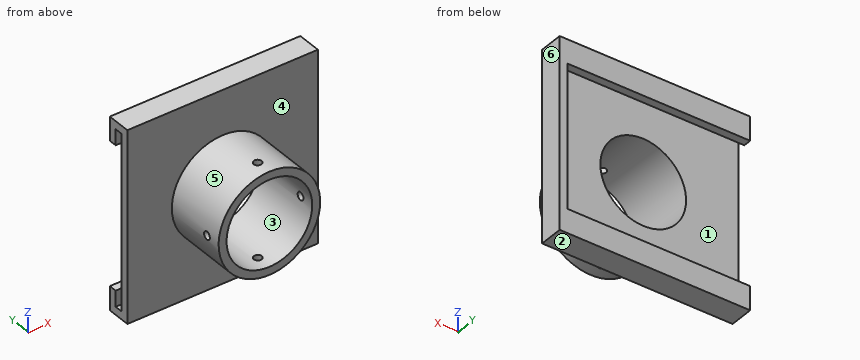
```python
from build123d import *

# Parameters (mm, degrees)
SKETCH1_R           = 20.32
SKETCH1_R_2         = 17.145
BOSS_EXTRUDE1_DEPTH = 25.4
SKETCH2_W           = 76.2
SKETCH2_H           = 76.2
SKETCH2_R           = 17.145
BOSS_EXTRUDE2_DEPTH = 3.175
SKETCH3_W           = 76.2
SKETCH3_H           = 3.175
BOSS_EXTRUDE3_DEPTH = 6.35
BOSS_EXTRUDE4_REACH = 91.465
SKETCH4_W           = 3.175
SKETCH4_H           = 6.35
SKETCH5_W           = 6.35
SKETCH5_H           = 3.175
BOSS_EXTRUDE5_DEPTH = 73.025
SKETCH7_R           = 1.5875
CUT_EXTRUDE1_DEPTH  = 65.210401221
CIRPATTERN1_COUNT   = 4


with BuildPart() as part:
    # Sketch1 → Boss-Extrude1 (new body)
    with BuildSketch(Plane(origin=(0, 0, 0), x_dir=(1, 0, 0), z_dir=(0, 1, 0))):
        with Locations(Location((0, 0, 0), (0, 0, 270))):
            Circle(SKETCH1_R)
        with Locations(Location((0, 0, 0), (0, 0, 270))):
            Circle(SKETCH1_R_2, mode=Mode.SUBTRACT)
    extrude(amount=BOSS_EXTRUDE1_DEPTH)

    # Sketch2 → Boss-Extrude2 (add)
    with BuildSketch(Plane(origin=(0, 25.4, 0), x_dir=(1, 0, 0), z_dir=(0, 1, 0))):
        Rectangle(SKETCH2_W, SKETCH2_H)
        with Locations(Location((0, 0, 0), (0, 0, 270))):
            Circle(SKETCH2_R, mode=Mode.SUBTRACT)
    extrude(amount=BOSS_EXTRUDE2_DEPTH)

    # Sketch3 → Boss-Extrude3 (add)
    with BuildSketch(Plane(origin=(0, 28.575, 0), x_dir=(1, 0, 0), z_dir=(0, 1, 0))):
        with Locations((0, 36.5125)):
            Rectangle(SKETCH3_W, SKETCH3_H)
        with Locations((0, -36.5125)):
            Rectangle(SKETCH3_W, SKETCH3_H)
    extrude(amount=BOSS_EXTRUDE3_DEPTH)

    # Sketch4 → Boss-Extrude4 (add, up to next)
    with BuildSketch(Plane.XY.offset(-34.925), mode=Mode.PRIVATE) as boss_extrude4_sk1:
        with Locations((36.5125, 31.75)):
            Rectangle(SKETCH4_W, SKETCH4_H)
    boss_extrude4_tool1 = extrude(boss_extrude4_sk1.sketch, amount=BOSS_EXTRUDE4_REACH, mode=Mode.PRIVATE) - part.part
    add(boss_extrude4_tool1.solids().sort_by_distance((36.5125, 31.75, -34.925))[0])

    # Sketch5 → Boss-Extrude5 (add)
    with BuildSketch(Plane.ZY.offset(-34.925)):
        with Locations((-31.75, 33.3375)):
            Rectangle(SKETCH5_W, SKETCH5_H)
        with Locations((31.75, 33.3375)):
            Rectangle(SKETCH5_W, SKETCH5_H)
    extrude(amount=BOSS_EXTRUDE5_DEPTH)

    # Sketch7 → Cut-Extrude1 (cut, symmetric)
    with BuildSketch(Plane(origin=(0, 0, 0), x_dir=(0, 0, -1), z_dir=(1, 0, 0))):
        with Locations((0, 6.35)):
            Circle(SKETCH7_R)
    cut_extrude1 = extrude(amount=CUT_EXTRUDE1_DEPTH, both=True, mode=Mode.SUBTRACT)

    # CirPattern1: Cut-Extrude1 ×4 about axis
    cirpattern1_axis = Axis((0, 25.4, 0), (0, -1, 0))
    for i in range(1, CIRPATTERN1_COUNT):
        add(cut_extrude1.rotate(cirpattern1_axis, i * 360 / CIRPATTERN1_COUNT), mode=Mode.SUBTRACT)


solid = part.part
```
Read the model definition and answer for the solid it produces. Units are mm, in the model's axes. Face numbers are marked on the shaded views. A direction names the side the tool comes from. Give positions to 0.01 mm unless a question says otherwise; leave off trailing zeros. Write each loop counter-clockwise with the first axis right and the second up, starting at its lowest first coordinate (ties: lowest second). Pieces come first, ordered by that corner, then holes. Notation, with made-up numbers: (84, 76) - (129, 76) arc R29 ccw to (129, 104) - close; hole circle Ø2 at (44, 67.25). An arc over 180 degrees is marked (long way). Write item = value, one per line. Start each with the question number.
Item 1: Find section C-C (y = 27). Give the vertices of the cut face in (x, z) (3 decimals).
Item 2: A tool of negligible diameter and unlimited length cuts with its end or side. For the marked faces 1 and 2, from which of +Z, -Z, +X, -X, +Y, -Y can it reach the whole face along a straight path? Write none if from no direction.
Item 3: The mould has two halves that part along X. Classify the marked faces 3, 4, 5 and 6: +X half, -X half, draft (parallel to the pull), parting line (faces both ways), or undercut.
Item 4: Each of these flat-tipped pins is pushed along its axis until it touches: P1, Ø1.5, axis at x = 3, z = 16.5, coming from the +Y side (3 decimals); P2, Ø2.5, axis at x = 0, y = 6.35, coming from the -Z side; P3, Ø1.9, axis at x = -4.5, z = 31, coming from the -Y side; P4, Ø10, axis at y = 6, z = 8.5, coming from the +X side. Where does it stop, or does it pass through?
Item 5: Find section D-D (z = -24). Give the vertices of the cut face in (x, y) (3 decimals), then the cut area to 3 significant figures.
Item 6: Find the intervals of material crossed by probe 1 along Z at (x, y) = (-17, 32) (3 decimals); probe 2 along Z at (x, y) = (0, 18) (3 decimals); probe 3 along Y at (x, z) = (17.85, 0) (1 decimal), in increasing order. Write a range as [from, to].
Item 7: Find section A-A (z = 0). Give the vertices of the cut face in (x, y) (1 decimal), then the cut area to 3 significant figures.
Item 8: Find section B-B (x = 0). State how many separate pieces and enclosed holes the cut face has, then the cut area to 3 significant figures.
Response:
q1.outline = (-38.1, -38.1) - (38.1, -38.1) - (38.1, 38.1) - (-38.1, 38.1) - close; hole circle Ø34.29 at (0, 0)
q2.face_1 = -X
q2.face_2 = -Z, +X, -X, +Y, -Y
q3.face_3 = undercut
q3.face_4 = draft
q3.face_5 = parting line
q3.face_6 = +X half
q4.P1 = 28.575
q4.P2 = through
q4.P3 = 25.4
q4.P4 = 20.02
q5.outline = (-38.1, 25.4) - (38.1, 25.4) - (38.1, 34.925) - (34.925, 34.925) - (34.925, 28.575) - (-38.1, 28.575) - close
q5.area = 262 mm²
q6.probe_1 = [-38.1, -28.575], [28.575, 38.1]
q6.probe_2 = [-20.32, -17.145], [17.145, 20.32]
q6.probe_3 = [0, 4.8], [7.9, 28.6]
q7.outline = (-38.1, 25.4) - (-20.3, 25.4) - (-20.3, 7.9) - (-17.1, 7.9) - (-17.1, 28.6) - (-38.1, 28.6) - close; (-20.3, 0) - (-17.1, 0) - (-17.1, 4.8) - (-20.3, 4.8) - close; (17.1, 0) - (20.3, 0) - (20.3, 4.8) - (17.1, 4.8) - close; (17.1, 7.9) - (20.3, 7.9) - (20.3, 25.4) - (38.1, 25.4) - (38.1, 34.9) - (34.9, 34.9) - (34.9, 28.6) - (17.1, 28.6) - close
q7.area = 294 mm²
q8.separate_pieces = 4
q8.enclosed_holes = 0
q8.area = 355 mm²
